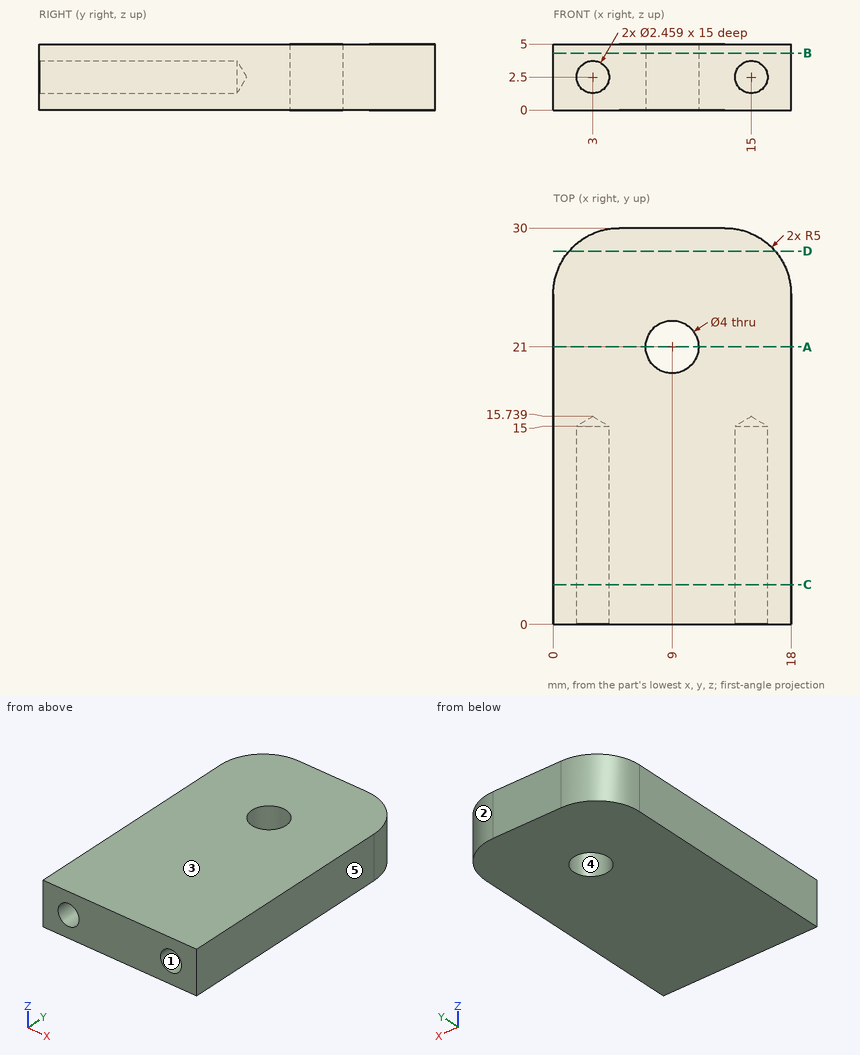
Here's the drawing with two shaded views (mm, measured from the low corner). I have some questions. A direction names the side the tool comes from. Round coordinates to 2 decimals unless told otherwise and drop trailing zeros. Loops run counter-clockwise (first coordinate to the right, second up) from the corner with the lowest first, then second, coordinate; pieces in that order, holes last. Notation, with made-up numbers: M -6.5,-21 L 32.5,-21 A22 cw 32.5,-6 Z; hole C 53.25,-30.5 d10. An arc over 180 degrees is marked long. Answer as a JSON object with one key per item and string values. Group by question number.
Q1. Please list where these lines run through material, in increasing order: L1, parallel to X at y = 7, z = 2.55; L2, parallel to Z at x = 15, y = 8; L3, parallel to Z at x = 15.75, y = 8.5 (1 decimal).
Q2. Imagine slicing it at B-B, the plane z = 4.3. Please give me the cut outline in (x, y), then the cut area to 3 significant figures.
Q3. On a 3-axis mill with a long thin cutter (end or side, diameter ignored), from which of +Z, -Z, +X, -X, +Y, -Y can I reach the whole of each face in a straight line? I mean the marked faces 1 and 2. Say none if no direction works.
Q4. We'd pull the mould along X, two halves only. Please class the marked faces 3, 4 and 5: +X half, -X half, draft (parallel to the pull), parting line (faces both ways), or undercut.
Q5. Imagine slicing it at A-A, the plane y = 21. Please give me the cut outline in (x, z).
Q6. Imagine slicing it at D-D, the plane y = 28.25. Please give me the cut outline in (x, z), then the cut area to 3 significant figures.
Q7. Will these pins go through, and if not, where does the flat tip stop? pin 1 (2 mm diameter, centred on x = 3, z = 2.5, fed in from -Y); pin 2 (1 mm diameter, centred on x = 5, z = 1.5, fed in from -Y).
Q8. Imagine slicing it at C-C, the plane y = 3. Please give me the cut outline in (x, z).
Findings:
{
 "1": {"L1": "x = 0 to 1.77, 4.23 to 13.77, 16.23 to 18", "L2": "z = 0 to 1.27, 3.73 to 5", "L3": "z = 0 to 1.5, 3.5 to 5"},
 "2": {"outline": "M 0,0 L 18,0 L 18,25 A5 ccw 13,30 L 5,30 A5 ccw 0,25 Z; hole C 9,21 d4", "area": "517 mm2"},
 "3": {"face 1": "-Y", "face 2": "+Z, -Z, +X, +Y"},
 "4": {"face 3": "draft", "face 4": "undercut", "face 5": "+X half"},
 "5": {"outline": "M 0,0 L 7,0 L 7,5 L 0,5 Z; M 11,0 L 18,0 L 18,5 L 11,5 Z"},
 "6": {"outline": "M 1.2,0 L 16.8,0 L 16.8,5 L 1.2,5 Z", "area": "78.0 mm2"},
 "7": {"pin 1": "stops at y = 15.14", "pin 2": "stops at y = 0"},
 "8": {"outline": "M 0,0 L 18,0 L 18,5 L 0,5 Z; hole C 3,2.5 d2.46; hole C 15,2.5 d2.46"}
}
